Here's how the part is built. I have some questions about the finished solid (model axes, mm). A direction names the side the tool comes from. Give positions to 0.01 mm unless a question says otherwise; leave off trailing zeros. Loops run counter-clockwise (first coordinate to the right, second up) from the corner with the lowest first, then second, coordinate; pieces in that order, holes last. Notation, with made-up numbers: (-27.75, 59) -> (22.25, 59) arc R18 cw to (22.25, 67) -> close; hole circle Ø2 at (21, 8.25). An arc over 180 degrees is marked (long way). Answer in a Markdown table with one row per item. Add a question column.
Item 1: If we section it at B-B (x = 26): Write out the boundary of the cut face in (y, z), then the cut area to 4 significant figures.
Item 2: Which directions (+Z, -Z, +X, -X, +Y, -Y) give clear straight access to the entire face, cutting with the end or side of a thin tool? Please do faces 1 (the face through (14, 0, -23)), 2 (the face through (26, 3, -5)), 3 (the face through (0, 3, -23)), 4 (the face through (1, 3, -5)).
Item 3: If we section it at D-D (x = 17): Write out the boundary of the cut face in (y, z), then the cut area to 3 significant figures.
Item 4: If we section it at A-A (z = -7): Write out the boundary of the cut face in (x, y), then the cut area to 3 significant figures.
Item 5: If I drill on line 1 (X direction, y = 2, z = -7); line 2 (Y direction, x = 21.5, z = -3.5); line 3 (Z direction, x = 15.5, y = -3.25), over which ranges is the centre line in solid material (lowest first)?
Item 6: We'd pull the mould along X, two halves only. Please class faces 5 (the face through (14, 3, -42)), 6 (the face through (3, 0, -2)), 7 (the face through (28, 3, -23)), 8 (the face through (25, 3, -7)): released by +X, released by -X, zero draft, split by the parting line, or undercut.
Item 7: If we section it at C-C (y = 4.25): Write out the boundary of the cut face in (x, z), then the cut area to 3 significant figures.
Item 8: For P1, Ø4, axis at y = -0.5, z = -3, coming from the -X side; P2, Ø2.5, axis at x = 26.5, y = 2, coming from the +Z side; P3, Ø3, axis at x = 9.5, y = -7, coming from the -Z side; P4, Ø8, axis at y = -7, z = -37, coming from the +X side, each with a flat end and sliding along its axis, tell me the tip position at first contact or that it passes through.
```python
from build123d import *

# Parameters (mm, degrees)
SKETCH2_W           = 28
SKETCH2_H           = 42
BOSS_EXTRUDE1_DEPTH = 5.5
SKETCH3_W           = 3
SKETCH3_H           = 5
CUT_EXTRUDE1_DEPTH  = 5.5
SKETCH4_W           = 22
SKETCH4_H           = 2.5
BOSS_EXTRUDE2_DEPTH = 10
SKETCH5_R           = 1
CUT_EXTRUDE2_DEPTH  = 10


with BuildPart() as part:
    # Sketch2 → Boss-Extrude1 (new body)
    with BuildSketch(Plane(origin=(0, 0, 0), x_dir=(1, 0, 0), z_dir=(0, 1, 0))):
        with Locations((14, 21)):
            Rectangle(SKETCH2_W, SKETCH2_H)
    extrude(amount=BOSS_EXTRUDE1_DEPTH)

    # Sketch3 → Cut-Extrude1 (cut)
    with BuildSketch(Plane(origin=(0, 5.5, 0), x_dir=(1, 0, 0), z_dir=(0, 1, 0))):
        with Locations((1.5, 2.5)):
            Rectangle(SKETCH3_W, SKETCH3_H)
        with Locations((26.5, 2.5)):
            Rectangle(SKETCH3_W, SKETCH3_H)
    extrude(amount=-CUT_EXTRUDE1_DEPTH, mode=Mode.SUBTRACT)

    # Sketch4 → Boss-Extrude2 (add)
    with BuildSketch(Plane.XZ):
        with Locations((14, -1.25)):
            Rectangle(SKETCH4_W, SKETCH4_H)
    extrude(amount=BOSS_EXTRUDE2_DEPTH)

    # Sketch5 → Cut-Extrude2 (cut)
    with BuildSketch(Plane(origin=(0, 5.5, 0), x_dir=(1, 0, 0), z_dir=(0, 1, 0))):
        with Locations(Location((2, 7, 0), (0, 0, 270))):
            Circle(SKETCH5_R)
        with Locations(Location((26, 7, 0), (0, 0, 270))):
            Circle(SKETCH5_R)
    extrude(amount=-CUT_EXTRUDE2_DEPTH, mode=Mode.SUBTRACT)


solid = part.part
```
Recorded:
| question | item | result |
|---|---|---|
| 1 | outline | (0, -42) -> (5.5, -42) -> (5.5, -8) -> (0, -8) -> close; (0, -6) -> (5.5, -6) -> (5.5, -5) -> (0, -5) -> close |
| 1 | area | 192.5 mm^2 |
| 2 | face 1 | -Z, +X, -X, -Y |
| 2 | face 2 | +Z, +X, +Y, -Y |
| 2 | face 3 | +Z, -Z, -X, +Y, -Y |
| 2 | face 4 | +Z, -X, +Y, -Y |
| 3 | outline | (-10, -2.5) -> (0, -2.5) -> (0, -42) -> (5.5, -42) -> (5.5, 0) -> (-10, 0) -> close |
| 3 | area | 256 mm^2 |
| 4 | outline | (0, 0) -> (1, 0) -> (1, 5.5) -> (0, 5.5) -> close; (3, 0) -> (25, 0) -> (25, 5.5) -> (3, 5.5) -> close; (27, 0) -> (28, 0) -> (28, 5.5) -> (27, 5.5) -> close |
| 4 | area | 132 mm^2 |
| 5 | line 1 | x = 0 to 1, 3 to 25, 27 to 28 |
| 5 | line 2 | y = 0 to 5.5 |
| 5 | line 3 | z = -2.5 to 0 |
| 6 | face 5 | zero draft |
| 6 | face 6 | released by -X |
| 6 | face 7 | released by +X |
| 6 | face 8 | undercut |
| 7 | outline | (0, -42) -> (28, -42) -> (28, -5) -> (25, -5) -> (25, 0) -> (3, 0) -> (3, -5) -> (0, -5) -> close; hole circle Ø2 at (2, -7); hole circle Ø2 at (26, -7) |
| 7 | area | 1,140 mm^2 |
| 8 | P1 | stops at x = 3 |
| 8 | P2 | stops at z = -5 |
| 8 | P3 | stops at z = -2.5 |
| 8 | P4 | passes through |
